Source: CAD feature listing. Evaluate the final solid. Frame: model axes, mm. Give positions to 0.01 mm unless a question says otherwise; leave off trailing zeros. Loops run counter-clockwise (first coordinate to the right, second up) from the corner with the lowest first, then second, coordinate; pieces in that order, holes last. Notation, with made-up numbers: M 2,50.25 L 13,50.25 A28 cw 13,70.25 Z; hole C 8,-31 d5. An arc over 180 degrees is marked long. Put each result on its own line as item: value.
from build123d import *

# Parameters (mm, degrees)
SKETCH1_W           = 20
SKETCH1_H           = 40
BOSS_EXTRUDE1_DEPTH = 2
SKETCH2_R           = 2
SKETCH2_R_2         = 0.5
CUT_EXTRUDE1_DEPTH  = 2


with BuildPart() as part:
    # Sketch1 → Boss-Extrude1 (new body)
    with BuildSketch(Plane(origin=(0, 0, 0), x_dir=(1, 0, 0), z_dir=(0, 1, 0))):
        Polygon((-14, -27.5), (-9, -27.5), (-9, -29.5), (-5, -29.5), (-5, -27.5), (5, -27.5), (5, -29.5), (9, -29.5), (9, -27.5), (14, -27.5), (14, 27.5), (9, 27.5), (9, 29.5), (5, 29.5), (5, 27.5), (-5, 27.5), (-5, 29.5), (-9, 29.5), (-9, 27.5), (-14, 27.5), (-14, 14.5), (-14, -14.5), align=None)
        Rectangle(SKETCH1_W, SKETCH1_H, mode=Mode.SUBTRACT)
    extrude(amount=BOSS_EXTRUDE1_DEPTH)

    # Sketch2 → Cut-Extrude1 (cut)
    with BuildSketch(Plane(origin=(0, 2, 0), x_dir=(1, 0, 0), z_dir=(0, 1, 0))):
        with Locations(Location((4.75, 24.25, 0), (0, 0, 270))):
            Circle(SKETCH2_R)
        with Locations(Location((-4.75, 24.25, 0), (0, 0, 90))):
            Circle(SKETCH2_R)
        with Locations(Location((4.75, -24.25, 0), (0, 0, 270))):
            Circle(SKETCH2_R)
        with Locations(Location((-4.75, -24.25, 0), (0, 0, 90))):
            Circle(SKETCH2_R)
        with Locations(Location((10, -24.01, 0), (0, 0, 270))):
            Circle(SKETCH2_R_2)
    extrude(amount=-CUT_EXTRUDE1_DEPTH, mode=Mode.SUBTRACT)


solid = part.part
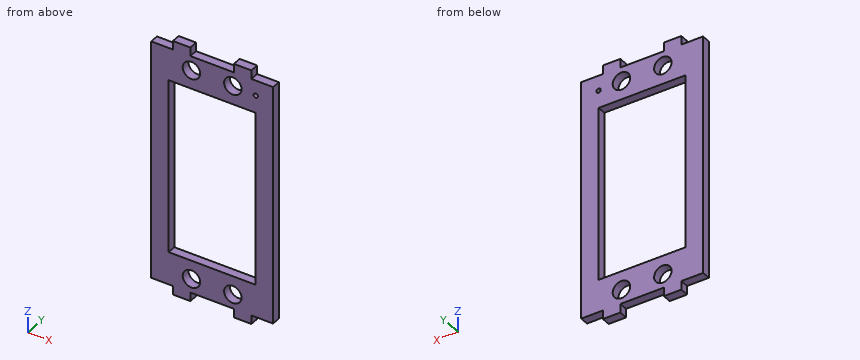
1. Section query D-D (z = -10.5). Output: boundary loops of the cut face in (x, y).
Found:
outline: M -14,0 L -10,0 L -10,2 L -14,2 Z; M 10,0 L 14,0 L 14,2 L 10,2 Z
2. Section query C-C (z = -24.25). Output: boundary loops of the cut face in (x, y), plus the area to 3 significant figures.
Found:
outline: M -14,0 L -6.75,0 L -6.75,2 L -14,2 Z; M -2.75,0 L 2.75,0 L 2.75,2 L -2.75,2 Z; M 6.75,0 L 14,0 L 14,2 L 6.75,2 Z
area: 40.0 mm^2
3. Section query A-A (x = -2). Output: boundary loops of the cut face in (y, z).
Found:
outline: M 0,-27.5 L 2,-27.5 L 2,-20 L 0,-20 Z; M 0,20 L 2,20 L 2,27.5 L 0,27.5 Z
4. Material intervals for line 1 (Z direction, x = -4.75, y = 1); line 2 (X direction, y = 1, z = -24.25); line 3 (X direction, y = 0.35, z = -2), sorted ascending. Write a range as from..to.
Found:
line 1: -27.5..-26.25, -22.25..-20, 20..22.25, 26.25..27.5
line 2: -14..-6.75, -2.75..2.75, 6.75..14
line 3: -14..-10, 10..14
5. Contact query for flat-ended pins moving along their axis: P1, Ø1, axis at y = 1, z = -28.5, coming from the +X side; P2, Ø1, axis at x = -0.5, y = 1.5, coming from the +Z side; P3, Ø0.6, axis at y = 1.5, z = 28.5, coming from the -X side. Output: stop coordinate, or through.
Found:
P1: x = 9
P2: z = 27.5
P3: x = -9
6. Section query B-B (y = 1.7). State how many separate pieces and enclosed holes the cut face has, plus the area to 3 significant figures.
Found:
separate pieces: 1
enclosed holes: 6
area: 721 mm^2
